Check sheet for the modelled part. Datum: model origin and axes. Units: mm. A direction names the side the tool comes from. Round coordinates to 2 decimals unless told otherwise and drop trailing zeros. Loops run counter-clockwise (first coordinate to the right, second up) from the corner with the lowest first, then second, coordinate; pieces in that order, holes last. Notation, with made-up numbers: (-24, -35.5) - (9, -35.5) arc R17 cw to (9, -24.5) - close; hole circle Ø5 at (67, 6.25). An arc over 180 degrees is marked (long way). Return JSON: item names as keys, results as strings.
from build123d import *

# Parameters (mm, degrees)
F0_W     = 15
F0_H     = 14.4
F1_DEPTH = 15
F2_R     = 13
F3_R     = 1.999218
F4_DEPTH = 8.5


with BuildPart() as f1:
    # F0 (on Right) → F1 (new body, symmetric)
    with BuildSketch(Plane.YZ):
        with Locations((7.5, 8.768751)):
            Rectangle(F0_W, F0_H)
    extrude(amount=F1_DEPTH, both=True)

    # F2
    f2_edges = [f1.edges().sort_by_distance(p)[0] for p in [
        (-15, 15, 8.768751),
        (15, 15, 8.768751),
    ]]
    fillet(f2_edges, radius=F2_R)

    # F3 (on face) → F4 (cut)
    with BuildSketch(Plane.XY.offset(15.968751)):
        with Locations((0, 7.5)):
            Circle(F3_R)
    extrude(amount=-F4_DEPTH, mode=Mode.SUBTRACT)


solid = f1.part
Q1. Sectioned sample at A-A (z = 10.5). Enter the section's corners in (x, y), plus the area to 3 significant figures.
Answer key:
{"outline": "(-15, 0) - (15, 0) - (15, 2) arc R13 ccw to (2, 15) - (-2, 15) arc R13 ccw to (-15, 2) - close; hole circle Ø4 at (0, 7.5)", "area": "365 mm²"}
Q2. Draft check along Y on faces 1 (the face through (-15, 1, 9)), 2 (the face through (0, 8, 7.469)), 3 (the face through (0, 15, 9)). Enter one of: released by +Y, released by -Y, zero draft, split by the parting line, or undercut.
Answer key:
{"face 1": "zero draft", "face 2": "undercut", "face 3": "released by +Y"}
Q3. Tool access check on faces 4 (the face through (-0.433, 5.548, 11.778)), 5 (the face through (0, 4, 15.969)). Record the directions out of +Z, -Z, +X, -X, +Y, -Y that give a thin tool (end or side, any length) a straight path to the whole face; none if there is none.
Answer key:
{"face 4": "+Z", "face 5": "+Z, +X, -X, +Y, -Y"}
Q4. Sectioned sample at B-B (x = 0). Enter the section's corners in (y, z).
Answer key:
{"outline": "(0, 1.57) - (15, 1.57) - (15, 15.97) - (9.5, 15.97) - (9.5, 7.47) - (5.5, 7.47) - (5.5, 15.97) - (0, 15.97) - close"}
Q5. Scan lines: probe 1 along Y at (x, z) = (0, 9.5); probe 2 along Y at (x, z) = (10, 5.25); probe 3 along X at (y, z) = (11.75, 13.75). Record each from-to range of solid material in increasing order. Write a range as [from, to].
Answer key:
{"probe 1": "y = [0, 5.5], [9.5, 15]", "probe 2": "y = [0, 12.25]", "probe 3": "x = [-10.6, 10.6]"}
Q6. Sectioned sample at D-D (y = 6.25). Enter the section's corners in (x, z).
Answer key:
{"outline": "(-14.29, 1.57) - (14.29, 1.57) - (14.29, 15.97) - (1.56, 15.97) - (1.56, 7.47) - (-1.56, 7.47) - (-1.56, 15.97) - (-14.29, 15.97) - close"}
Q7. Depth check by flat-ended pin: P1, Ø6, axis at x = 4.5, z = 13.5, coming from the +Y side; P2, Ø1.5, axis at y = 5, z = 3.5, coming from the -X side; P3, Ø3, axis at y = 10, z = 3.5, coming from the -X side; P4, Ø8, axis at y = 10, z = 10.5, coming from the +X side. Enter the tip coordinate at first touch or a pass-through.
Answer key:
{"P1": "stops at y = 15", "P2": "stops at x = -14.8", "P3": "stops at x = -13.26", "P4": "stops at x = 14.37"}
Q8. Sectioned sample at C-C (z = 3.5). Enter the section's corners in (x, y).
Answer key:
{"outline": "(-15, 0) - (15, 0) - (15, 2) arc R13 ccw to (2, 15) - (-2, 15) arc R13 ccw to (-15, 2) - close"}
